Source: CAD feature listing. Evaluate the final solid. Frame: model axes, mm. A direction names the side the tool comes from. Coordinates: 2 decimals unless noted, no trailing zeros. Loops run counter-clockwise (first coordinate to the right, second up) from the corner with the lowest first, then second, coordinate; pieces in that order, holes last.
from build123d import *

# Parameters (mm, degrees)
F0_R     = 162
F0_R_2   = 157.0000052452
F1_DEPTH = 2200
F2_R     = 30.15
F3_DEPTH = 163.000000104
F4_R     = 30.15
F5_DEPTH = 163.0000001
F6_DEPTH = 163.0000001
F7_DEPTH = 163.000000104


with BuildPart() as f1:
    # F0 (on Front) → F1 (new body)
    with BuildSketch(Plane.XZ):
        Circle(F0_R)
        Circle(F0_R_2, mode=Mode.SUBTRACT)
    extrude(amount=F1_DEPTH)

    # F2 (on Top) → F3 (cut, up to face)
    with BuildSketch(Plane.XY):
        with Locations((0, -50)):
            Circle(F2_R)
    extrude(amount=F3_DEPTH, mode=Mode.SUBTRACT)

    # F4 (on Right) → F5 (cut, up to face)
    with BuildSketch(Plane.YZ):
        with Locations((-150, 0)):
            Circle(F4_R)
    extrude(amount=F5_DEPTH, mode=Mode.SUBTRACT)

    # F4 (on Right) → F6 (cut, up to face)
    with BuildSketch(Plane.YZ):
        with Locations((-2050, 0)):
            Circle(F4_R)
    extrude(amount=-F6_DEPTH, mode=Mode.SUBTRACT)

    # F2 (on Top) → F7 (cut, up to face)
    with BuildSketch(Plane.XY):
        with Locations((0, -2150)):
            Circle(F2_R)
    extrude(amount=-F7_DEPTH, mode=Mode.SUBTRACT)


solid = f1.part
Q1. Draft query along X for faces 5 (the cylindrical face through (149.75, -1084.6, 47.16)), 6 (the flat face through (-133, -2200, 85)), 7 (the cylindrical face through (154.52, -1084.6, 48.66)). Return one class per face: +X half, -X half, draft (parallel to the pull), parting line (faces both ways), or undercut.
Q2. Section B-B, the plane x = 0. Return the cut outline in (y, z), plus the area to 3 significant figures.
Q3. Section D-D, the plane x = 111. Return the cut outline in (y, z), plus the area to 3 significant figures.
Q4. Contact query for flat-ended pins moving along their axis: pin 1 Ø6 at (x, y) = (96, -1832.5) entering from -Z; pin 2 Ø4 at (y, z) = (-261, 87.5) entering from -X; pin 3 Ø3 at (y, z) = (-463, -30.5) entering from -X. Output: stop coordinate, or through.
Q5. Access query for faces 1 (the cylindrical face through (-157.98, -2080.12, 1.33)), 2 (the cylindrical face through (-22.2, -29.6, 158)), 3 (the cylindrical face through (-22.2, -2129.6, -158)), 4 (the cylindrical face through (157.98, -180.12, 1.33)). Directions: +Z, -Z, +X, -X, +Y, -Y. A direction counts if a zero-diameter tool reaches every point of the face in a straight line with its end or side. Return the directions, or none.
Q6. Section C-C, the plane z = 129. Return the cut outline in (x, y), plus the area to 3 significant figures.
Q7. Line query: line 1 along X through (y, z) = (-1420, 0); line 2 along Y through (x, z) = (0, 157.75); line 3 along Z through (x, y) = (6, -456). Output: solid intervals per line, ascending.
Q8. Section A-A, the plane z = 0. Return the cut outline in (x, y), plus the area to 3 significant figures.
Derived:
1. face 5: undercut
1. face 6: draft
1. face 7: parting line
2. outline: (-2200, -162) - (-2180.15, -162) - (-2180.15, -157) - (-2200, -157) - close; (-2200, 157) - (-80.15, 157) - (-80.15, 162) - (-2200, 162) - close; (-2119.85, -162) - (0, -162) - (0, -157) - (-2119.85, -157) - close; (-19.85, 157) - (0, 157) - (0, 162) - (-19.85, 162) - close
2. area: 21,400 mm2
3. outline: (-2200, -118) - (0, -118) - (0, -111.03) - (-2200, -111.03) - close; (-2200, 111.03) - (0, 111.03) - (0, 118) - (-2200, 118) - close
3. area: 30,600 mm2
4. pin 1: stops at z = -132.65
4. pin 2: stops at x = -137.6
4. pin 3: stops at x = -159.38
5. face 1: -X
5. face 2: +Z
5. face 3: -Z
5. face 4: +X
6. outline: (-97.99, -2200) - (-89.49, -2200) - (-89.49, 0) - (-97.99, 0) - close; (89.49, -2200) - (97.99, -2200) - (97.99, 0) - (89.49, 0) - close
6. area: 37,400 mm2
7. line 1: x = -162 to -157, 157 to 162
7. line 2: y = -2200 to -80.15, -19.85 to 0
7. line 3: z = -161.89 to -156.89, 156.89 to 161.89
8. outline: (-162, -2200) - (-157, -2200) - (-157, -2080.15) - (-162, -2080.15) - close; (-162, -2019.85) - (-157, -2019.85) - (-157, 0) - (-162, 0) - close; (157, -2200) - (162, -2200) - (162, -180.15) - (157, -180.15) - close; (157, -119.85) - (162, -119.85) - (162, 0) - (157, 0) - close
8. area: 21,400 mm2
